Here's the drawing with two shaded views (mm, measured from the low corner). I have some questions. Give positions to 0.01 mm unless a question says otherwise; leave off trailing zeros. Loops run counter-clockwise (first coordinate to the right, second up) from the corner with the lowest first, then second, coordinate; pieces in that order, holes last. Notation, with made-up numbers: (-31.5, 11) - (2.5, 11) arc R23 ccw to (2.5, 40) - close; hole circle Ø4 at (-16, -36.5). An arc over 180 degrees is marked (long way). Use one line per item in the form item = value.
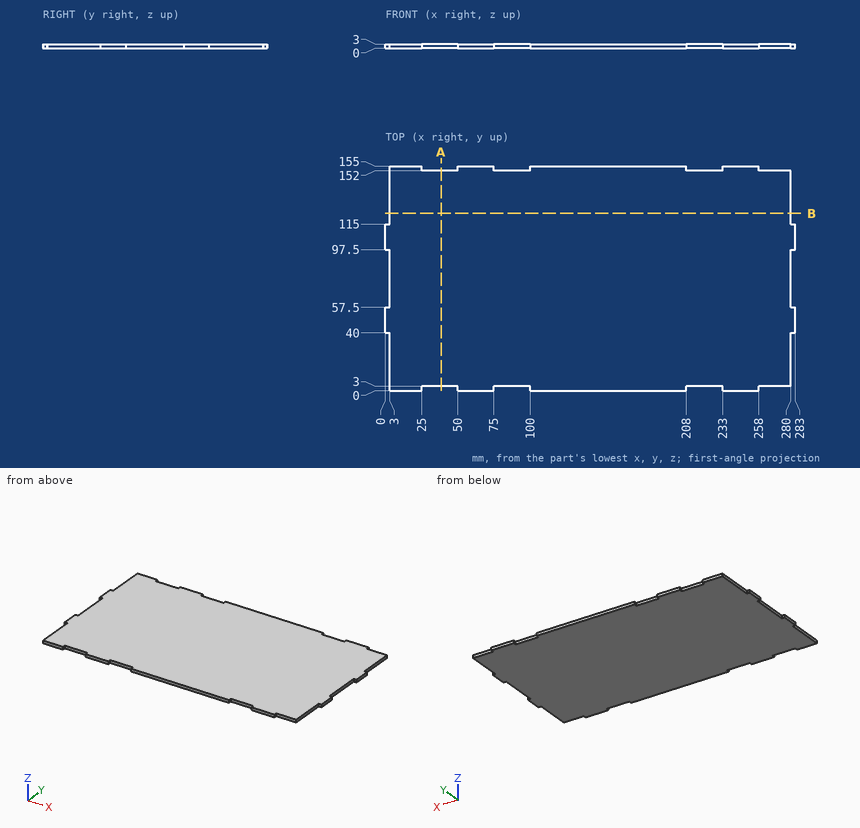
(1) If I drill on probe 1 along Y at (x, z) = (259, 0.5); probe 2 along X at (y, z) = (39, 0.95), over which ranges is the centre line in solid material (lowest first)?
Geometry says:
probe_1 = 3 to 152
probe_2 = 3 to 280
(2) If we section it at A-A (x = 38.5): List the corners of the cut face in (y, z) for me, plus the area to 3 significant figures.
Geometry says:
outline = (3, 0) - (152, 0) - (152, 3) - (3, 3) - close
area = 447 mm²
(3) For P1, Ø1.5, axis at y = 23, z = 1.5, coming from the +X side; P2, Ø0.9, axis at y = 153, z = 1, coming from the +X side; P3, Ø0.9, axis at y = 2, z = 1, coming from the -X side; P4, Ø5, axis at x = 155.5, y = 23.5, coming from the -Z side, each with a flat end and sliding along its axis, tell me the tip position at first contact or that it passes through.
Geometry says:
P1 = 280
P2 = 258
P3 = 3
P4 = 0
(4) If we section it at B-B (y = 122.5): List the corners of the cut face in (x, z) for me, plus the area to 3 significant figures.
Geometry says:
outline = (3, 0) - (280, 0) - (280, 3) - (3, 3) - close
area = 831 mm²
